For this review, take the finished solid that the model builds, in its own axes (mm). A direction names the side the tool comes from. Give positions to 0.01 mm unless a question says otherwise; leave off trailing zeros. Order: outer loops, then holes, each group sorted by start corner. A loop starts at its lowest first (then second) coordinate and runs counter-clockwise, first axis right, second up.
Item 1: Consider section A-A (y = 1.3). Give the boundary of the cut face in (x, z).
Item 2: Consider section C-C (x = -5.25). Give the boundary of the cut face in (y, z), plus the area to 3 significant figures.
Item 3: For probe 1 along Y at (x, z) = (-3.25, 2); probe 2 along X at (y, z) = (3.15, 2.75); probe 3 along Y at (x, z) = (-6.5, 7.25), list the stretches that pass through material, from the lowest coordinate up.
Item 4: For P1, Ø1, axis at y = 2.5, z = 4.5, coming from the -X side; P2, Ø0.5, axis at x = -0.5, y = 1.5, coming from the +Z side; P3, Ø2.5, axis at x = -6.5, z = 4.5, coming from the +Y side, all flat-tipped, find the tip position at first contact; note any pin that passes through.
Item 5: Machinability: for faces 4 (the flat face through (-1.2, 3, 8)), 5 (the flat face through (-2.5, 3, 3)), 6 (the cylindrical face through (-1.902, 2.588, 7.31)), 7 (the flat face through (-2, 4, 10.2)), 8 (the flat face through (-7.8, 4.7, 3)), which of the approach directions +Z, -Z, +X, -X, +Y, -Y give a long, thin tool a straight path to every point of the face, cutting with its end or side? Answer none if there is none.
Item 6: Consider section B-B (z = 5). Give the boundary of the cut face in (x, y).
Item 7: The part is to be moulded in two halves that separate along Y. For faces 1 (the flat face through (-1, 3, 6.5)), 2 (the flat face through (-4, 0, 5)), 3 (the flat face through (-6, 2, 5.3)), say which applies: released by +Y, released by -Y, zero draft, split by the parting line, or undercut.
Item 8: Consider section D-D (y = 4.85). Give the boundary of the cut face in (x, z).
```python
from build123d import *

# Parameters (mm, degrees)
SKETCH_1_W                = 7.8
SKETCH_1_H                = 10.2
EXTRUDE_1_DEPTH           = 4.5
CUT_EXTRUDE_1_DEPTH       = 4
SKETCH_3_W                = 4.5
SKETCH_3_H                = 4
CUT_EXTRUDE_2_DEPTH       = 4.3
SKETCH_4_W                = 7.8
SKETCH_4_H                = 10.2
EXTRUDE_2_DEPTH           = 0.5
SKETCH_5_W                = 1.2
SKETCH_5_H                = 3.7
CUT_EXTRUDE_3_DEPTH       = 14.779695207
CUT_EXTRUDE_4_REACH       = 15.78
SKETCH_7_W                = 0.3
SKETCH_7_H                = 6.4
EXTRUDE_3_DEPTH           = 0.25
DRAFT_1_ANGLE             = -21.801409486
HOLE_WIZARD_4_0_4_1_D     = 4
HOLE_WIZARD_4_0_4_1_DEPTH = 5.7
CHAMFER_1_SIZE            = 1.2
CHAMFER_1_SIZE2           = 3.7
FILLET_1_R                = 0.2


with BuildPart() as part:
    # Эскиз1 → Бобышка-Вытянуть1 (new body)
    with BuildSketch(Plane(origin=(0, 5, 0), x_dir=(1, 0, 0), z_dir=(0, 1, 0))):
        with Locations((-3.9, -5.1)):
            Rectangle(SKETCH_1_W, SKETCH_1_H)
    extrude(amount=-EXTRUDE_1_DEPTH)

    # Эскиз2 → Вырез-Вытянуть1 (cut)
    with BuildSketch(Plane.XZ.offset(-0.5)):
        Polygon((-6.8, 0.8), (-6.8, 5.3), (-7.8, 6.3), (-7.8, 0.8), align=None)
    extrude(amount=-CUT_EXTRUDE_1_DEPTH, mode=Mode.SUBTRACT)

    # Эскиз3 → Вырез-Вытянуть2 (cut)
    with BuildSketch(Plane.ZY.offset(6.8)):
        with Locations((3.05, 2.5)):
            Rectangle(SKETCH_3_W, SKETCH_3_H)
    extrude(amount=-CUT_EXTRUDE_2_DEPTH, mode=Mode.SUBTRACT)

    # Эскиз4 → Бобышка-Вытянуть2 (add)
    with BuildSketch(Plane.XZ.offset(-0.5)):
        with Locations((-3.9, 5.1)):
            Rectangle(SKETCH_4_W, SKETCH_4_H)
    extrude(amount=EXTRUDE_2_DEPTH)

    # Эскиз5 → Вырез-Вытянуть3 (cut, through all)
    with BuildSketch(Plane(origin=(0, 5, 0), x_dir=(-1, 0, 0), z_dir=(0, 1, 0))):
        with Locations((0.6, 8.35)):
            Rectangle(SKETCH_5_W, SKETCH_5_H)
    extrude(amount=-CUT_EXTRUDE_3_DEPTH, mode=Mode.SUBTRACT)

    # Эскиз6 → Вырез-Вытянуть4 (cut, up to next)
    with BuildSketch(Plane(origin=(0, 0, 0), x_dir=(-1, 0, 0), z_dir=(0, 0, -1)), mode=Mode.PRIVATE) as cut_extrude_4_sk1:
        with BuildLine():
            Line((7.8, 2.1), (7.8, 2.9))
            Line((7.8, 2.9), (3.71823341, 2.9))
            ThreePointArc((3.71823341, 2.9), (3.31823341, 2.5), (3.71823341, 2.1))
            Line((3.71823341, 2.1), (7.8, 2.1))
        make_face()
    cut_extrude_4_tool1 = extrude(cut_extrude_4_sk1.sketch, amount=-CUT_EXTRUDE_4_REACH, mode=Mode.PRIVATE) & part.part
    add(cut_extrude_4_tool1.solids().sort_by_distance((-5.60113, 2.5, 0))[0], mode=Mode.SUBTRACT)

    # Эскиз7 → Бобышка-Вытянуть3 (add)
    with BuildSketch(Plane(origin=(0, 5, 0), x_dir=(-1, 0, 0), z_dir=(0, 1, 0))):
        with Locations((1.4, 3.2)):
            Rectangle(SKETCH_7_W, SKETCH_7_H)
    extrude(amount=EXTRUDE_3_DEPTH)

    # Уклон1
    draft_1_faces = [part.faces().sort_by_distance(p)[0] for p in [
        (-1.55, 5.125, 3.2),
        (-1.25, 5.125, 3.2),
    ]]
    draft(draft_1_faces, Plane.ZX.offset(5), DRAFT_1_ANGLE)

    # Диаметр отверстия Ø4.0 (4)1
    with Locations(Plane.XY.offset(10.2)):
        with Locations((-3.9, 2.5)):
            Hole(HOLE_WIZARD_4_0_4_1_D / 2, depth=HOLE_WIZARD_4_0_4_1_DEPTH)

    # Фаска1
    chamfer_1_edges = [part.edges().sort_by_distance(p)[0] for p in [
        (-7.8, 2.5, 10.2),
    ]]
    chamfer_1_side = [part.faces().sort_by_distance(p)[0] for p in [
        (-4.5, 4.917199034, 10.2),
    ]]
    chamfer(chamfer_1_edges, length=CHAMFER_1_SIZE, length2=CHAMFER_1_SIZE2, reference=chamfer_1_side[0])

    # Скругление1
    fillet_1_edges = [part.edges().sort_by_distance(p)[0] for p in [
        (0, 2.5, 6.5),
    ]]
    fillet(fillet_1_edges, radius=FILLET_1_R)


solid = part.part
```
Resolved:
1. outline: (-7.8, 0) - (0, 0) - (0, 6.3) arc R0.2 ccw to (-0.2, 6.5) - (-1.2, 6.5) - (-1.2, 10.2) - (-2.3, 10.2) - (-2.3, 4.5) - (-2.5, 4.5) - (-2.5, 0.8) - (-7.8, 0.8) - close; (-7.8, 6.3) - (-6.8, 5.3) - (-5.5, 5.3) - (-5.5, 10.2) - (-6.6, 10.2) - (-7.8, 6.5) - close
2. outline: (0, 0) - (2.1, 0) - (2.1, 0.8) - (0.5, 0.8) - (0.5, 5.3) - (1.02, 5.3) - (1.02, 10.2) - (0, 10.2) - close; (2.9, 0) - (5, 0) - (5, 10.2) - (3.98, 10.2) - (3.98, 5.3) - (4.5, 5.3) - (4.5, 0.8) - (2.9, 0.8) - close
2. area: 17.9 mm2
3. probe 1: y = 0 to 0.5, 4.5 to 5
3. probe 2: x = -2.5 to 0
3. probe 3: y = 0 to 5
4. P1: stops at x = -2.5
4. P2: stops at z = 6.5
4. P3: stops at y = 5
5. face 4: +Z, +X, +Y, -Y
5. face 5: -X
5. face 6: +Z
5. face 7: +Z, +X, -X, +Y, -Y
5. face 8: +Z, -Z, -X, +Y, -Y
6. outline: (-7.8, 0) - (0, 0) - (0, 5) - (-1.25, 5) - (-1.15, 5.25) - (-1.65, 5.25) - (-1.55, 5) - (-7.8, 5) - (-7.8, 4.5) - (-2.5, 4.5) - (-2.5, 3.93) arc R2 cw to (-2.5, 1.07) - (-2.5, 0.5) - (-7.8, 0.5) - close
7. face 1: zero draft
7. face 2: released by -Y
7. face 3: undercut
8. outline: (-7.8, 0) - (0, 0) - (0, 6.3) arc R0.2 ccw to (-0.2, 6.5) - (-1.2, 6.5) - (-1.2, 10.2) - (-6.6, 10.2) - (-7.8, 6.5) - close
